Could you check a few things on this model? Use its own coordinates, in mm. Coordinates: 2 decimals unless noted, no trailing zeros. Order: outer loops, then holes, each group sorted by start corner. A loop starts at its lowest first (then second) coordinate and runs counter-clockwise, first axis right, second up.
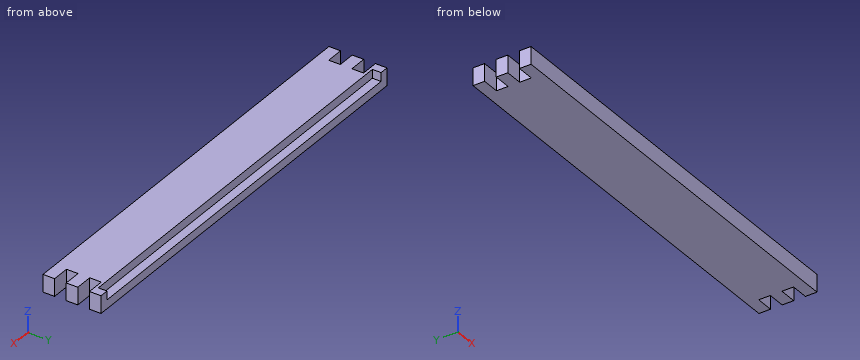
Autodesk Inventor part; units mm, degrees
ref_plane "YZ Plane" through (0, 0, 0) normal (1, 0, 0) x (0, 1, 0)
ref_plane "XZ Plane" through (0, 0, 0) normal (0, 1, 0) x (-1, 0, 0)
ref_plane "XY Plane" through (0, 0, 0) normal (0, 0, 1) x (1, 0, 0)
sketch "Sketch1" plane through (0, 0, 0) normal (0, 0, 1) x (1, 0, 0)
  line L0 (293.6875, 89.6306) -> (523.875, 89.6306)
  line L1 (523.875, 89.6306) -> (523.875, 26.1306)
  line L2 (523.875, 26.1306) -> (293.6875, 26.1306)
  line L3 (293.6875, 89.6306) -> (293.6875, 76.9306)
  line L4 (293.6875, 76.9306) -> (274.6375, 76.9306)
  line L5 (274.6375, 76.9306) -> (274.6375, 64.2306)
  line L6 (274.6375, 64.2306) -> (293.6875, 64.2306)
  line L7 (293.6875, 64.2306) -> (293.6875, 51.5306)
  line L8 (293.6875, 51.5306) -> (274.6375, 51.5306)
  line L9 (274.6375, 51.5306) -> (274.6375, 38.8306)
  line L10 (274.6375, 38.8306) -> (293.6875, 38.8306)
  line L11 (293.6875, 38.8306) -> (293.6875, 26.1306)
  line L12 (293.6875, 76.9306) -> (312.7375, 76.9306)
  line L13 (312.7375, 76.9306) -> (312.7375, 64.2306)
  line L14 (312.7375, 64.2306) -> (293.6875, 64.2306)
  line L15 (293.6875, 51.5306) -> (312.7375, 51.5306)
  line L16 (312.7375, 51.5306) -> (312.7375, 38.8306)
  line L17 (312.7375, 38.8306) -> (293.6875, 38.8306)
  point P0 (0, 0)
  dimension "d4" = 63.5
  dimension "d17" = 230.1875
  dimension "d18" = 19.05
  dimension "d19" = 12.7
  dimension "d20" = 12.7
  dimension "d21" = 12.7
  dimension "d22" = 12.7
  dimension "d23" = 12.7
  dimension "d24" = 0
  dimension "d28" = 0
extrude "Extrusion4" add sketch "Sketch1" along normal blind 19.05 contours L0 L1 L2 L11 L17 L16 L15 L7 L14 L13 L12 L3
mirror "Mirror2" about plane through (523.875, 26.1306, 0) normal (1, 0, 0) of "Extrusion4"
sketch "Sketch4" plane through (293.6875, 89.6306, 19.05) normal (0, 1, 0) x (1, 0, 0)
  line L0 (0, 19.05) -> (0, 0)
  line L1 (0, 0) -> (460.375, 0)
  line L2 (460.375, 19.05) -> (460.375, 0)
  line L3 (9.525, 0) -> (450.85, 0)
  line L4 (450.85, 0) -> (450.85, 9.525)
  line L5 (450.85, 9.525) -> (9.525, 9.525)
  line L6 (9.525, 9.525) -> (9.525, 0)
  point P0 (-293.6875, 19.05)
  dimension "d32" = 9.525
  dimension "d34" = 9.525
extrude "Extrusion5" cut sketch "Sketch4" against normal blind 9.525
properties part number "top_cover_side" material "Wood (Birch)"
Item 1: Suppose I cut it at A-A (x = 720.5). List the corners of the cut face in (y, z) for me (3 decimals), and give its area (3 significant figures).
Item 2: For pin 1 Ø6.5 at (y, z) = (69.5, 11) entering from -X; pin 2 Ø7.5 at (x, z) = (542.5, 15) entering from +Y; pin 3 Ø10 at (y, z) = (49, 14) entering from -X; pin 4 Ø5 at (x, y) = (465.5, 87) entering from +Z (3 decimals), each with a flat end and sliding along its axis, tell me the tip position at first contact or that it passes through.
Item 3: I need wall thicknesses on line 1 (X direction, y = 87, z = 13.5); line 2 (X direction, y = 74, z = 4.75); line 3 (Y direction, x = 394, z = 12.5). Which ranges of each line are inside material? Lowest first, please.
Geometry results:
1. outline: (26.131, 0) - (89.631, 0) - (89.631, 9.525) - (80.106, 9.525) - (80.106, 19.05) - (26.131, 19.05) - close
1. area: 1,120 mm2
2. pin 1: stops at x = 312.74
2. pin 2: stops at y = 80.11
2. pin 3: stops at x = 293.69
2. pin 4: stops at z = 9.525
3. line 1: x = 293.69 to 303.21, 744.54 to 754.06
3. line 2: x = 312.74 to 735.01
3. line 3: y = 26.13 to 80.11
